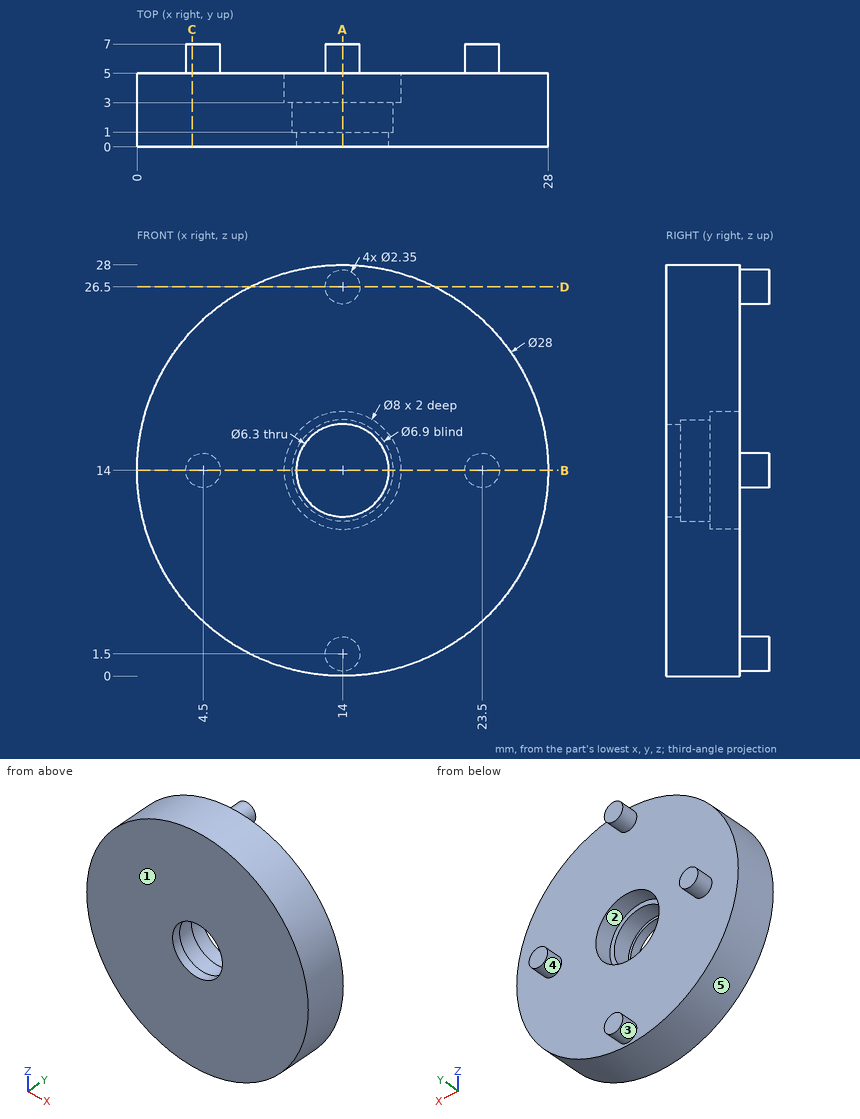
Input: dimensioned drawing with shaded views. Units: mm. Origin: part minimum x, y, z. A direction names the side the tool comes from. Coordinates: 2 decimals unless noted, no trailing zeros. Write each loop counter-clockwise with the first axis right and the second up, starting at its lowest first coordinate (ties: lowest second). Pieces come first, ordered by that corner, then holes. Notation, with made-up numbers: (48, 28.5) -> (76, 28.5) arc R12 ccw to (76, 42.5) -> close; hole circle Ø1 at (61, 9.25). An arc over 180 degrees is marked (long way). Return JSON: item names as keys, results as strings. Group by question number.
1) Section query B-B, the plane z = 14. Return loops of the section in (x, y) (3 decimals), plus the area to 3 significant figures.
2) Set-up query: the marked faces 4 and 5. Return all of +Z, -Z, +X, -X, +Y, -Y with unobstructed straight access to the full face (end or side cutting, diameter ignored); none if empty.
3) Section query D-D, the plane z = 26.5. Return loops of the section in (x, y) (3 decimals), plus the area to 3 significant figures.
4) Contact query for flat-ended pins moving along their axis: P1, Ø4, axis at y = 4.5, z = 24.5, coming from the -X side; P2, Ø8.5, axis at x = 15.5, z = 14, coming from the +Y side; P3, Ø3.5, axis at x = 12.5, z = 13.5, coming from the +Y side. Output: stop coordinate, or through.
5) Ray query, line 1 along X through (y, z) = (3.7, 14); line 2 along Z through (x, y) = (14, 2.05). Return the intervals inside material, ascending.
6) Mould query, pull axis X, two halves, no side actions, for the marked faces 1, 2 and 3. Classes: +X half, -X half, draft (parallel to the pull), parting line (faces both ways), or undercut.
7) Section query A-A, the plane x = 14. Return loops of the section in (y, z) (3 decimals).
8) Section query C-C, the plane x = 3.75. Return loops of the section in (y, z), plus the area to 3 significant figures.
From the geometry:
{
 "1": {"outline": "(0, 0) -> (10.85, 0) -> (10.85, 1) -> (10.55, 1) -> (10.55, 3) -> (10, 3) -> (10, 5) -> (5.675, 5) -> (5.675, 7) -> (3.325, 7) -> (3.325, 5) -> (0, 5) -> close; (17.15, 0) -> (28, 0) -> (28, 5) -> (24.675, 5) -> (24.675, 7) -> (22.325, 7) -> (22.325, 5) -> (18, 5) -> (18, 3) -> (17.45, 3) -> (17.45, 1) -> (17.15, 1) -> close", "area": "113 mm²"},
 "2": {"face 4": "+Y", "face 5": "+Y, -Y"},
 "3": {"outline": "(7.695, 0) -> (20.305, 0) -> (20.305, 5) -> (15.175, 5) -> (15.175, 7) -> (12.825, 7) -> (12.825, 5) -> (7.695, 5) -> close", "area": "67.7 mm²"},
 "4": {"P1": "x = 2.88", "P2": "y = 5", "P3": "y = 1"},
 "5": {"line 1": "0 to 10, 18 to 28", "line 2": "0 to 10.55, 17.45 to 28"},
 "6": {"face 1": "draft", "face 2": "undercut", "face 3": "parting line"},
 "7": {"outline": "(0, 0) -> (5, 0) -> (5, 0.325) -> (7, 0.325) -> (7, 2.675) -> (5, 2.675) -> (5, 10) -> (3, 10) -> (3, 10.55) -> (1, 10.55) -> (1, 10.85) -> (0, 10.85) -> close; (0, 17.15) -> (1, 17.15) -> (1, 17.45) -> (3, 17.45) -> (3, 18) -> (5, 18) -> (5, 25.325) -> (7, 25.325) -> (7, 27.675) -> (5, 27.675) -> (5, 28) -> (0, 28) -> close"},
 "8": {"outline": "(0, 4.46) -> (5, 4.46) -> (5, 13.1) -> (7, 13.1) -> (7, 14.9) -> (5, 14.9) -> (5, 23.54) -> (0, 23.54) -> close", "area": "99.0 mm²"}
}
